```python
from build123d import *

# Parameters (mm, degrees)
BOSS_EXTRUDE1_DEPTH   = 6.1722
SKETCH1_R             = 6.35
SKETCH1_R_2           = 4.7498
BOSS_EXTRUDE1_2_DEPTH = 6.1722
SKETCH2_R             = 6.35
BOSS_EXTRUDE2_DEPTH   = 1.778
SKETCH3_R             = 3.048
BOSS_EXTRUDE3_DEPTH   = 25.4
CUT_EXTRUDE1_START    = -25.4
CUT_EXTRUDE1_DEPTH    = 25.4
FILLET1_R             = 1.27
CUT_EXTRUDE2_DEPTH    = 2.54


with BuildPart() as part:
    # Sketch1 → Boss-Extrude1 (new body)
    with BuildSketch(Plane.XY):
        Polygon((-2.413, 1.3931462), (-2.413, -1.3931462), (0, -2.786292399), (2.413, -1.3931462), (2.413, 1.3931462), (0, 2.786292399), align=None)
    extrude(amount=BOSS_EXTRUDE1_DEPTH)



with BuildPart() as body_2:
    # Sketch1 → Boss-Extrude1 2 (new body)
    with BuildSketch(Plane.XY):
        Circle(SKETCH1_R)
        Circle(SKETCH1_R_2, mode=Mode.SUBTRACT)
    extrude(amount=BOSS_EXTRUDE1_2_DEPTH)


with BuildPart() as part_1:
    add(part.part)

    add(body_2.part)  # Boss-Extrude2 merges body 2
    # Sketch2 → Boss-Extrude2 (add)
    with BuildSketch(Plane.XY.offset(6.1722)):
        Circle(SKETCH2_R)
    extrude(amount=BOSS_EXTRUDE2_DEPTH)

    # Sketch3 → Boss-Extrude3 (add)
    with BuildSketch(Plane.XY.offset(7.9502)):
        with Locations(Location((0, 0, 0), (0, 0, 180))):
            Circle(SKETCH3_R)
    extrude(amount=BOSS_EXTRUDE3_DEPTH)

    # Sketch4 → Cut-Extrude1 (cut)
    with BuildSketch(Plane.XY.offset(33.3502).offset(CUT_EXTRUDE1_START)):
        with BuildLine():
            Line((2.093142983, 2.215639062), (2.093142983, -2.215639062))
            ThreePointArc((2.093142983, -2.215639062), (3.048, 0), (2.093142983, 2.215639062))
        make_face()
    extrude(amount=CUT_EXTRUDE1_DEPTH, mode=Mode.SUBTRACT)

    # Fillet1
    fillet1_edges = [part_1.edges().sort_by_distance(p)[0] for p in [
        (-3.048, 0, 7.9502),
        (2.093142983, 0, 7.9502),
    ]]
    fillet(fillet1_edges, radius=FILLET1_R)

    # Sketch5 → Cut-Extrude2 (cut)
    with BuildSketch(Plane(origin=(0, 0, 0), x_dir=(-1, 0, 0), z_dir=(0, 0, -1))):
        Polygon((2.413, -1.3931462), (2.413, 1.3931462), (0, 2.786292399), (-2.413, 1.3931462), (-2.413, -1.3931462), (0, -2.786292399), align=None)
    extrude(amount=-CUT_EXTRUDE2_DEPTH, mode=Mode.SUBTRACT)


solid = part_1.part
```
Geometry: final body of the model. Coordinates: model frame, mm. A direction names the side the tool comes from. Give positions to 0.01 mm unless a question says otherwise; leave off trailing zeros. Loops run counter-clockwise (first coordinate to the right, second up) from the corner with the lowest first, then second, coordinate; pieces in that order, holes last. Notation, with made-up numbers: (84, 47.25) - (122, 47.25) arc R34 cw to (122, 77.25) - close; hole circle Ø6 at (45, -11). An arc over 180 degrees is marked (long way). Answer as CSV lines item,"result". Start each with the question number.
(1) Mould query, pull axis X, two halves, no side actions, for faces 4 (the face through (2.093, 0, 21)), 5 (the face through (1, -5, 0)), 6 (the face through (-2.413, 0, 4)). Classes: +X half, -X half, draft (parallel to the pull), parting line (faces both ways), or undercut.
(2) Reachability of faces 1 (the face through (4, 0, 7.95)), 2 (the face through (0, 0, 33.35)), 3 (the face through (-1.19, 2.1, 4.33)) from +Z, -Z, +X, -X, +Y, -Y: full face, straight path, thin tool, end or side. Return the list, or none.
(3) Section query B-B (z = 14). Output: boundary loops of the cut face in (x, y), and give its area (3 significant figures).
(4) Pin query (flat end, axial travel): P1, Ø1, axis at x = 4, y = -1.5, coming from the +Z side; P2, Ø4, axis at x = 1, y = 1, coming from the -Z side; P3, Ø1.3, axis at y = -1, z = 26, coming from the +X side; P4, Ø2, axis at x = -5, z = 9.5, coming from the -Y side. Return the tip coordinate at first contact, or that it passes through.
(5) Section query A-A (z = 5.5). Output: boundary loops of the cut face in (x, y), and give its area (3 significant figures).
(6) Section query C-C (x = 5.25). Output: boundary loops of the cut face in (y, z).
(7) Ray query, line 1 along Y through (x, z) = (0, 2.5); line 2 along X through (y, z) = (0.75, 3); line 3 along Z through (x, y) = (3.25, -5). Return the intervals inside material, ascending. Write a range as [from, to].
Worked answers:
1,face 4,"+X half"
1,face 5,"draft"
1,face 6,"undercut"
2,face 1,"+Z"
2,face 2,"+Z, +X, -X, +Y, -Y"
2,face 3,"-Z"
3,outline,"(2.09, -2.22) - (2.09, 2.22) arc R3.05 ccw (long way) to start"
3,area,"26.3 mm^2"
4,P1,"stops at z = 7.95"
4,P2,"stops at z = 2.54"
4,P3,"stops at x = 2.09"
4,P4,"passes through"
5,outline,"circle Ø12.7 at (0, 0); (-2.41, -1.39) - (0, -2.79) - (2.41, -1.39) - (2.41, 1.39) - (0, 2.79) - (-2.41, 1.39) - close; hole circle Ø9.5 at (0, 0)"
5,area,"76.0 mm^2"
6,outline,"(-3.57, 0) - (3.57, 0) - (3.57, 7.95) - (-3.57, 7.95) - close"
7,line 1,"y = [-6.35, -4.75], [4.75, 6.35]"
7,line 2,"x = [-6.31, -4.69], [-2.41, 2.41], [4.69, 6.31]"
7,line 3,"z = [0, 7.95]"
